Autodesk Inventor part; units mm, degrees
ref_plane "YZ Plane" through (0, 0, 0) normal (1, 0, 0) x (0, 1, 0)
ref_plane "XZ Plane" through (0, 0, 0) normal (0, 1, 0) x (-1, 0, 0)
ref_plane "XY Plane" through (0, 0, 0) normal (0, 0, 1) x (1, 0, 0)
sketch "Sketch1" plane through (0, 0, 0) normal (0, 1, 0) x (-1, 0, 0)
  circle A0 centre (0, 0) radius 10
  circle A1 centre (0, 0) radius 5
  line L0 (8, 0) -> (8, -6)
  line L1 (2, -4.5826) -> (2, -9.798)
  line L2 (10, 0) -> (5, 0)
  line L3 (7.0711, 7.0711) -> (-7.0711, -7.0711) construction
  line L4 (0, 8) -> (-6, 8)
  line L5 (-4.5826, 2) -> (-9.798, 2)
  line L6 (0, 10) -> (0, 5)
  line L7 (10, 0) -> (10, -9.798)
  line L8 (10, -9.798) -> (2, -9.798)
  line L9 (0, 10) -> (-9.798, 10)
  line L10 (-9.798, 10) -> (-9.798, 2)
  line L11 (-4.5826, 2) -> (0, 2)
  line L12 (0, 2) -> (0, 5)
  line L13 (5, 0) -> (2, 0)
  line L14 (2, 0) -> (2, -4.5826)
  line L15 (-6, 8) -> (-9.798, 8)
  line L16 (8, -6) -> (8, -9.798)
  line L17 (-3.345, 2) -> (-3.345, 9.4239)
  line L18 (2, -3.345) -> (9.4239, -3.345)
  point P0 (-9.798, 2)
  point P1 (8, -3.345)
  point P2 (-3.345, 8)
  point P3 (-9.798, 2)
  dimension "d0" = 20
  dimension "d1" = 10
  dimension "d10" = 6
  dimension "d11" = 2
  dimension "d12" = 45
  dimension "d15" = 3.3451
extrude "Extrusion1" add sketch "Sketch1" along normal blind 95 contours L2 A1 L6 A0 | L7 L8 L16 A0 | A0 L18 L0 L2 | L6 L4 L17 A0 | A0 L15 L10 L9 | A0 L0 L18 | L0 L18 A1 L2 | L17 L4 A0 | L6 A1 L17 L4 | L13 L14 A1 L11 L12 | A1 L18 L14 L13 | L12 L11 L17 A1 | A0 L5 A1 L1
extrude "Extrusion2" cut sketch "Sketch1" along normal blind 20 contours L2 A1 L6 A0 | L7 L8 L16 A0 | A0 L18 L0 L2 | L6 L4 L17 A0 | A0 L15 L10 L9 | A0 L0 L18 | L0 L18 A1 L2 | L17 L4 A0 | L6 A1 L17 L4 | A0 L1 A1 L18 L0 | L4 L17 A1 L5 A0 | A0 L10 L15 | A0 L5 A1 L1
extrude "Extrusion3" add sketch "Sketch1" along normal blind 20 contours A1 L18 L14 L13 | L12 L11 L17 A1 | A1 L14 L18 | L17 L11 A1
sketch "Sketch2" plane through (0, 95, 0) normal (0, 1, 0) x (1, 0, 0)
  line L0 (-10, 9.798) -> (-10, 0)
  line L1 (0, -10) -> (9.798, -10)
  point P0 (0, 0)
  point P1 (-3, -3)
  dimension "d16" = 7
  dimension "d24" = 7
hole "Hole1" at (-3, 95, 3) direction (0, -1, 0) diameter 4 depth 7 countersink diameter 4.2 countersink angle 90
sketch "Sketch3" plane through (0, 0, 0) normal (0, -1, 0) x (1, 0, 0)
  circle A0 centre (0, 0) radius 5
hole "Hole2" at (0, 0, 0) direction (0, 1, 0) diameter 4 depth 7 countersink diameter 4.2 countersink angle 90
properties part number "filar(5)" material "ABS Plastic"
CAD build for the part. Positions are in the model's coordinates, mm. A direction names the side the tool comes from. Round coordinates to 2 decimals unless told otherwise and drop trailing zeros. Loops run counter-clockwise (first coordinate to the right, second up) from the corner with the lowest first, then second, coordinate; pieces in that order, holes last. Notation, with made-up numbers: (26, 30.25) - (53, 30.25) arc R24 cw to (53, 47.25) - close; hole circle Ø3 at (-22, 14). An arc over 180 degrees is marked (long way). Return JSON: item names as keys, results as strings. Group by question number.
Q1. Band-saw the part on C-C on z = 6.75. Give the cut face in (x, y) (3 decimals), plus the area to 3 significant figures.
Q2. Band-saw the part on B-B on y = 60. Give the cut face in (x, z) (3 decimals), plus the area to 3 significant figures.
Q3. Flat gauge pins, fed straight in: pin 1 Ø3 at (x, z) = (3.5, -8) entering from -Y; pin 2 Ø8 at (y, z) = (29.5, -4.5) entering from +X; pin 3 Ø6.5 at (x, y) = (-6.5, 67.5) entering from -Z. Where does each tip first touch, or does it go through?
Q4. Two-plate mould, pull along Z, no slides. Class faces 1 (the face through (-2.2, 0, -1)), 2 (the face through (-1, 91, 3)), 3 (the face through (-9, 57, -9.798)), 4 (the face through (2, 4, 0)): +Z half, -Z half, draft (parallel to the pull), parting line (faces both ways), or undercut.
Q5. Drill centre lines: line 1 along Z through (x, y) = (6, 64); line 2 along Z through (x, y) = (0, 3.25). Where is each one in solid material? Low to high. Write a range as [from, to].
Q6. Band-saw the part on A-A on z = -8.5. Give the cut face in (x, y).
Q7. Tool access for faces 5 (the face through (9.798, 57, 9)), 6 (the face through (7, 57, 8)), 7 (the face through (7, 57, 2)), 8 (the face through (-3.505, 9.86, -3.566)): list every direction of +Z, -Z, +X, -X, +Y, -Y with a clear straight run to the whole face (end or side of a thin tool).
Solutions:
{
 "1": {"outline": "(-7.378, 20) - (3.345, 20) - (3.345, 95) - (-7.378, 95) - close", "area": "804 mm^2"},
 "2": {"outline": "(-10, -9.798) - (-8, -9.798) - (-8, -3.345) - (-2, -3.345) - (-2, -9.798) arc R10 ccw to (9.798, 2) - (3.345, 2) - (3.345, 8) - (9.798, 8) - (9.798, 10) - (0, 10) arc R10 ccw to (-10, 0) - close", "area": "276 mm^2"},
 "3": {"pin 1": "stops at y = 20", "pin 2": "stops at x = 9.99", "pin 3": "stops at z = -9.8"},
 "4": {"face 1": "draft", "face 2": "undercut", "face 3": "-Z half", "face 4": "undercut"},
 "5": {"line 1": "z = [-8, 2], [8, 10]", "line 2": "z = [-5, -2], [2, 5]"},
 "6": {"outline": "(-10, 20) - (-8, 20) - (-8, 95) - (-10, 95) - close; (-2, 20) - (5.27, 20) - (5.27, 95) - (-2, 95) - close"},
 "7": {"face 5": "+Z, +X, +Y, -Y", "face 6": "+X, +Y, -Y", "face 7": "+X, +Y", "face 8": "-Y"}
}
